from build123d import *

# Parameters (mm, degrees)
SKETCH1_W           = 35
SKETCH1_H           = 70
SKETCH1_R           = 1
SKETCH1_W_2         = 22
SKETCH1_H_2         = 44
BOSS_EXTRUDE1_DEPTH = 2.5
BOSS_EXTRUDE2_START = -2.5
BOSS_EXTRUDE2_DEPTH = 5


with BuildPart() as part:
    # Sketch1 → Boss-Extrude1 (new, symmetric)
    with BuildSketch(Plane(origin=(0, 0, 0), x_dir=(0, 0, -1), z_dir=(1, 0, 0))):
        with Locations((0, -6)):
            Rectangle(SKETCH1_W, SKETCH1_H)
        with Locations((-4.85, -24)):
            Circle(SKETCH1_R, mode=Mode.SUBTRACT)
        with Locations((4.85, -24)):
            Circle(SKETCH1_R, mode=Mode.SUBTRACT)
        with Locations((4.85, 24)):
            Circle(SKETCH1_R, mode=Mode.SUBTRACT)
        with Locations((-4.85, 24)):
            Circle(SKETCH1_R, mode=Mode.SUBTRACT)
        Rectangle(SKETCH1_W_2, SKETCH1_H_2, mode=Mode.SUBTRACT)
    extrude(amount=BOSS_EXTRUDE1_DEPTH, both=True)

    # Sketch2 → Boss-Extrude2 (add)
    with BuildSketch(Plane(origin=(0, 0, 0), x_dir=(0, 0, -1), z_dir=(1, 0, 0)).offset(BOSS_EXTRUDE2_START)):
        Polygon((17.5, -41), (17.5, -56), (10, -56), (10, -48.5), (-10, -48.5), (-10, -108.5), (25, -108.5), (25, -99), (32.5, -99), (32.5, -116), (-17.5, -116), (-17.5, -41), align=None)
    extrude(amount=BOSS_EXTRUDE2_DEPTH)


solid = part.part
Input: part model. Units: mm. Frame: model coordinates. A direction names the side the tool comes from. Give positions to 0.01 mm unless a question says otherwise; leave off trailing zeros. Order: outer loops, then holes, each group sorted by start corner. A loop starts at its lowest first (then second) coordinate and runs counter-clockwise, first axis right, second up. Notation, with made-up numbers: M 62.5,40 L 114.5,40 A26 cw 114.5,75 Z; hole C 73,20 d6. An arc over 180 degrees is marked long. Answer as a JSON object with one key per item and string values.
1. Reachability of faces 1 (the flat face through (0, -116, -8)), 2 (the flat face through (0, -48.5, 0)), 3 (the flat face through (0, -104, -25)) from +Z, -Z, +X, -X, +Y, -Y: full face, straight path, thin tool, end or side. Return the list, or none.
Result sheet:
{"face 1": "+Z, -Z, +X, -X, -Y", "face 2": "+X, -X", "face 3": "+X, -X, +Y"}
2. Ray query, line 1 (Y direction, x = -0.2, z = -4.85); line 2 (Z direction, x = 1.45, y = -10); line 3 (Z direction, x = -1.25, y = -55). Return the intervals inside material, ascending. Write a range as [from, to].
Result sheet:
{"line 1": "[-116, -108.5], [-48.5, -25], [-23, -22], [22, 23], [25, 29]", "line 2": "[-17.5, -11], [11, 17.5]", "line 3": "[-17.5, -10], [10, 17.5]"}
3. Cut plane A-A, the plane y = -19. Output: boundary loops of the cut face in (x, z).
Result sheet:
{"outline": "M -2.5,-17.5 L 2.5,-17.5 L 2.5,-11 L -2.5,-11 Z; M -2.5,11 L 2.5,11 L 2.5,17.5 L -2.5,17.5 Z"}
4. Cut plane C-C, the plane x = -0.9. Output: boundary loops of the cut face in (y, z), and give its area (3 significant figures).
Result sheet:
{"outline": "M -116,-32.5 L -99,-32.5 L -99,-25 L -108.5,-25 L -108.5,10 L -48.5,10 L -48.5,-10 L -56,-10 L -56,-17.5 L 29,-17.5 L 29,17.5 L -116,17.5 Z; hole C -24,-4.85 d2; hole C -24,4.85 d2; hole M -22,-11 L 22,-11 L 22,11 L -22,11 Z; hole C 24,-4.85 d2; hole C 24,4.85 d2", "area": "2,680 mm²"}
5. Pull-direction query (Y, two-part tool) for faces 4 (the flat face through (0, -99, -29)), 5 (the flat face through (0, -56, -14)), 6 (the flat face through (0, -13, -17.5)), 7 (the flat face through (0, 0, -11)); classes: +Y half, -Y half, draft (parallel to the pull), parting line (faces both ways), or undercut.
Result sheet:
{"face 4": "+Y half", "face 5": "undercut", "face 6": "draft", "face 7": "undercut"}
6. Cut plane B-B, the plane z = -14.5. Output: boundary loops of the cut face in (x, y).
Result sheet:
{"outline": "M -2.5,-116 L 2.5,-116 L 2.5,-108.5 L -2.5,-108.5 Z; M -2.5,-56 L 2.5,-56 L 2.5,29 L -2.5,29 Z"}
7. Cut plane D-D, the plane y = -85. Output: boundary loops of the cut face in (x, z), and give its area (3 significant figures).
Result sheet:
{"outline": "M -2.5,10 L 2.5,10 L 2.5,17.5 L -2.5,17.5 Z", "area": "37.5 mm²"}
